```python
from build123d import *

# Parameters (mm, degrees)
SKETCH_1_W          = 56
SKETCH_1_H          = 23.5
SKETCH_1_R          = 0.6
EXTRUDE_1_DEPTH     = 3
SKETCH_2_R          = 0.75
CUT_EXTRUDE_1_DEPTH = 37.67764987
SKETCH_2_3_R        = 1.5
SKETCH_2_3_R_2      = 0.75
CUT_EXTRUDE_2_DEPTH = 1.2
CUT_EXTRUDE_START   = -22.3
SKETCH_2_4_R        = 1.5
SKETCH_2_4_R_2      = 0.75
CUT_EXTRUDE_3_DEPTH = 1.2
SKETCH_3_W          = 22.5
SKETCH_3_H          = 10
SKETCH_3_W_2        = 10
SKETCH_3_H_2        = 34
EXTRUDE_2_DEPTH     = 12.4
SKETCH_4_R          = 0.6
CUT_EXTRUDE_4_DEPTH = 2
SKETCH_5_W          = 84.5
SKETCH_5_H          = 26
SKETCH_5_W_2        = 4.2
SKETCH_5_H_2        = 15.1
CUT_EXTRUDE_5_DEPTH = 9.4


with BuildPart() as part:
    # 草图1 → 凸台-拉伸1 (new body)
    with BuildSketch(Plane(origin=(0, 0, 0), x_dir=(1, 0, 0), z_dir=(0, 1, 0))):
        Rectangle(SKETCH_1_W, SKETCH_1_H)
        with Locations(Location((-20, 9.25, 0), (0, 0, 270))):
            Circle(SKETCH_1_R, mode=Mode.SUBTRACT)
        with Locations(Location((-20, -9.25, 0), (0, 0, 270))):
            Circle(SKETCH_1_R, mode=Mode.SUBTRACT)
        with Locations(Location((20, 9.25, 0), (0, 0, 270))):
            Circle(SKETCH_1_R, mode=Mode.SUBTRACT)
        with Locations(Location((20, -9.25, 0), (0, 0, 270))):
            Circle(SKETCH_1_R, mode=Mode.SUBTRACT)
    extrude(amount=EXTRUDE_1_DEPTH)

    # 草图2 → 切除-拉伸1 (cut, through all)
    with BuildSketch(Plane.XY.offset(11.75)):
        with Locations((-25, 0)):
            Circle(SKETCH_2_R)
        with Locations((25, 0)):
            Circle(SKETCH_2_R)
    extrude(amount=-CUT_EXTRUDE_1_DEPTH, mode=Mode.SUBTRACT)

    # 草图2<3> → 切除-拉伸2 (cut)
    # profile 1 of 2: a face of its own
    with BuildSketch(Plane.XY.offset(11.75)):
        with Locations((-25, 0)):
            Circle(SKETCH_2_3_R)
        with Locations((-25, 0)):
            Circle(SKETCH_2_3_R_2, mode=Mode.SUBTRACT)
    # profile 2 of 2: a face of its own
    with BuildSketch(Plane.XY.offset(11.75)):
        with Locations((25, 0)):
            Circle(SKETCH_2_3_R)
        with Locations((25, 0)):
            Circle(SKETCH_2_3_R_2, mode=Mode.SUBTRACT)
    extrude(amount=-CUT_EXTRUDE_2_DEPTH, mode=Mode.SUBTRACT)

    # 草图2<4> → 切除-拉伸3 (cut)
    # profile 1 of 2: a face of its own
    with BuildSketch(Plane.XY.offset(11.75).offset(CUT_EXTRUDE_START)):
        with Locations((-25, 0)):
            Circle(SKETCH_2_4_R)
        with Locations((-25, 0)):
            Circle(SKETCH_2_4_R_2, mode=Mode.SUBTRACT)
    # profile 2 of 2: a face of its own
    with BuildSketch(Plane.XY.offset(11.75).offset(CUT_EXTRUDE_START)):
        with Locations((25, 0)):
            Circle(SKETCH_2_4_R)
        with Locations((25, 0)):
            Circle(SKETCH_2_4_R_2, mode=Mode.SUBTRACT)
    extrude(amount=-CUT_EXTRUDE_3_DEPTH, mode=Mode.SUBTRACT)

    # 草图3 → 凸台-拉伸2 (add)
    with BuildSketch(Plane.XZ):
        with Locations((-39.25, 0)):
            Rectangle(SKETCH_3_W, SKETCH_3_H)
        with Locations((39.25, 0)):
            Rectangle(SKETCH_3_W, SKETCH_3_H)
        Rectangle(SKETCH_3_W_2, SKETCH_3_H_2)
    extrude(amount=-EXTRUDE_2_DEPTH)

    # 草图4 → 切除-拉伸4 (cut)
    with BuildSketch(Plane(origin=(0, 12.4, 0), x_dir=(1, 0, 0), z_dir=(0, 1, 0))):
        with Locations(Location((0, 15, 0), (0, 0, 270))):
            Circle(SKETCH_4_R)
        with Locations(Location((0, -15, 0), (0, 0, 270))):
            Circle(SKETCH_4_R)
        with Locations(Location((49, 0, 0), (0, 0, 270))):
            Circle(SKETCH_4_R)
        with Locations(Location((-49, 0, 0), (0, 0, 270))):
            Circle(SKETCH_4_R)
    extrude(amount=-CUT_EXTRUDE_4_DEPTH, mode=Mode.SUBTRACT)

    # 草图5 → 切除-拉伸5 (cut)
    with BuildSketch(Plane(origin=(0, 12.4, 0), x_dir=(1, 0, 0), z_dir=(0, 1, 0))):
        with Locations((-0.55, 0)):
            Rectangle(SKETCH_5_W, SKETCH_5_H)
        with Locations((-44.9, 0.45)):
            Rectangle(SKETCH_5_W_2, SKETCH_5_H_2)
    extrude(amount=-CUT_EXTRUDE_5_DEPTH, mode=Mode.SUBTRACT)


solid = part.part
```
Verification items for the finished model (mm, model axes). A direction names the side the tool comes from. Coordinates: 2 decimals unless noted, no trailing zeros. Loops run counter-clockwise (first coordinate to the right, second up) from the corner with the lowest first, then second, coordinate; pieces in that order, holes last. Notation, with made-up numbers: (33, 70) -> (48, 70) arc R38 cw to (48, 109) -> close; hole circle Ø4 at (-15, 16.25). An arc over 180 degrees is marked (long way). Put each result on its own line as item: value.
1. Section check B-B, the plane y = 6. Record the boundary of the cut face in (x, z).
Result set:
outline: (-50.5, -5) -> (-47, -5) -> (-47, 5) -> (-50.5, 5) -> close; (-5, -17) -> (5, -17) -> (5, -13) -> (-5, -13) -> close; (-5, 13) -> (5, 13) -> (5, 17) -> (-5, 17) -> close; (41.7, -5) -> (50.5, -5) -> (50.5, 5) -> (41.7, 5) -> close
2. Gauge pin test, flat ends, axial feed: P1, Ø6, axis at x = -34, y = 5.5, coming from the -Z side; P2, Ø3.5, axis at x = -19, y = 1.5, coming from the -Z side; P3, Ø0.9, axis at y = 1, z = 7.5, coming from the -X side. Record the tip position at first contact, or that the pin passes through.
Result set:
P1: stops at z = -5
P2: stops at z = -11.75
P3: stops at x = -28
3. Section check D-D, the plane z = 7.5. Record the boundary of the cut face in (x, y), then the cut area to 3 significant figures.
Result set:
outline: (-28, 0) -> (-25.75, 0) arc R0.75 cw to (-24.25, 0) -> (24.25, 0) arc R0.75 cw to (25.75, 0) -> (28, 0) -> (28, 3) -> (-28, 3) -> close
area: 166 mm^2
4. Section check C-C, the plane z = 2. Record the boundary of the cut face in (x, y).
Result set:
outline: (-50.5, 0) -> (-25.75, 0) arc R0.75 cw to (-24.25, 0) -> (24.25, 0) arc R0.75 cw to (25.75, 0) -> (50.5, 0) -> (50.5, 12.4) -> (41.7, 12.4) -> (41.7, 3) -> (-47, 3) -> (-47, 12.4) -> (-50.5, 12.4) -> close
5. Tool access check on faces 1 (the face through (44, 5, -5)), 2 (the face through (0, 8, 13)), 3 (the face through (5, 6, 15)), 4 (the face through (-5, 6, 15)). Record the directions out of +Z, -Z, +X, -X, +Y, -Y that give a thin tool (end or side, any length) a straight path to the whole face; none if there is none.
Result set:
face 1: -Z, +X, +Y, -Y
face 2: +X, -X, +Y
face 3: +Z, +X, +Y, -Y
face 4: +Z, -X, +Y, -Y
6. Mould release check, pull along Z, two halves, no side actions. Record for faces 5 (the face through (0, 8, -13)), 6 (the face through (5, 6, -15)), 7 (the face through (44, 5, 5)), 8 (the face through (0, 6, -17)): pulls with the +Z half, pulls with the -Z half, needs draft (parallel to the pull), parting line crosses it, or undercut.
Result set:
face 5: undercut
face 6: needs draft
face 7: pulls with the +Z half
face 8: pulls with the -Z half
7. Section check A-A, the plane y = 11.5. Record the boundary of the cut face in (x, z).
Result set:
outline: (-50.5, -5) -> (-47, -5) -> (-47, 5) -> (-50.5, 5) -> close; (-5, -17) -> (5, -17) -> (5, -13) -> (-5, -13) -> close; (-5, 13) -> (5, 13) -> (5, 17) -> (-5, 17) -> close; (41.7, -5) -> (50.5, -5) -> (50.5, 5) -> (41.7, 5) -> close; hole circle Ø1.2 at (-49, 0); hole circle Ø1.2 at (0, -15); hole circle Ø1.2 at (0, 15); hole circle Ø1.2 at (49, 0)
8. Thickness scan on line 1 (X direction, y = 2.1, z = -9.25); line 2 (Z direction, x = -49, y = 11.75); line 3 (Z direction, x = -3, y = 12). Record the ranges inside material, lowest first.
Result set:
line 1: x = -28 to -20.6, -19.4 to 19.4, 20.6 to 28
line 2: z = -5 to -0.6, 0.6 to 5
line 3: z = -17 to -13, 13 to 17
